Can you work these out from the model? Positions are in its coordinate system, mm. A direction names the side the tool comes from. Coordinates: 2 decimals unless noted, no trailing zeros. Loops run counter-clockwise (first coordinate to the right, second up) from the corner with the lowest first, then second, coordinate; pieces in that order, holes last. Notation, with made-up numbers: M 57.5,27 L 74.5,27 A11 cw 74.5,47 Z; hole C 33.25,70 d6. An arc over 180 degrees is marked long. Return JSON: item names as keys, results as strings. Group by question number.
```python
from build123d import *

# Parameters (mm, degrees)
SKETCH1_W           = 30
SKETCH1_H           = 30
SKETCH1_W_2         = 26
SKETCH1_H_2         = 26
BOSS_EXTRUDE1_DEPTH = 800
SKETCH2_W           = 30
SKETCH2_H           = 30
SKETCH2_R           = 11
BOSS_EXTRUDE2_DEPTH = 10
BOSS_EXTRUDE3_START = -10
SKETCH3_W           = 30
SKETCH3_H           = 30
SKETCH3_R           = 11
BOSS_EXTRUDE3_DEPTH = 10
SKETCH4_R           = 11
CUT_EXTRUDE1_DEPTH  = 50


with BuildPart() as part:
    # Sketch1 → Boss-Extrude1 (new body)
    with BuildSketch(Plane.XY):
        Rectangle(SKETCH1_W, SKETCH1_H)
        Rectangle(SKETCH1_W_2, SKETCH1_H_2, mode=Mode.SUBTRACT)
    extrude(amount=BOSS_EXTRUDE1_DEPTH)

    # Sketch2 → Boss-Extrude2 (add)
    with BuildSketch(Plane(origin=(0, 0, 0), x_dir=(-1, 0, 0), z_dir=(0, 0, -1))):
        with Locations((0, 30)):
            Rectangle(SKETCH2_W, SKETCH2_H)
        with Locations((0, 30)):
            Circle(SKETCH2_R, mode=Mode.SUBTRACT)
    extrude(amount=-BOSS_EXTRUDE2_DEPTH)

    # Sketch3 → Boss-Extrude3 (add)
    with BuildSketch(Plane.XY.offset(800).offset(BOSS_EXTRUDE3_START)):
        with Locations((0, 30)):
            Rectangle(SKETCH3_W, SKETCH3_H)
        with Locations(Location((0, 30, 0), (0, 0, 180))):
            Circle(SKETCH3_R, mode=Mode.SUBTRACT)
    extrude(amount=BOSS_EXTRUDE3_DEPTH)

    # Sketch4 → Cut-Extrude1 (cut)
    with BuildSketch(Plane.XZ.offset(15)):
        with Locations(Location((0, 400, 0), (0, 0, 270))):
            Circle(SKETCH4_R)
    extrude(amount=-CUT_EXTRUDE1_DEPTH, mode=Mode.SUBTRACT)


solid = part.part
```
1) For pin 1 (6 mm diameter, centred on x = -9, y = 34.5, fed in from +Z); pin 2 (9 mm diameter, centred on x = 0, y = 24.5, fed in from +Z); pin 3 (12 mm diameter, centred on x = -8.5, z = 528, fed in from +Y), each with a flat end and sliding along its axis, tell me the tip position at first contact or that it passes through.
2) Suppose I cut it at C-C, the plane z = 400. List the corners of the cut face in (x, y) for me.
3) If we mould it in two halves opening along X, with no side actions, what happens to faces 4 (the face through (-10, 15, 395)), 5 (the face through (-15, 1, 394)), 6 (the face through (15, 1, 394)), 7 (the face through (2.38, 19.26, 4.93))? For each: +X half, -X half, draft (parallel to the pull), parting line (faces both ways), or undercut.
4) If I drill on line 1 (Y direction, x = 0, z = 796.25); line 2 (Y direction, x = -0.5, z = 493.5), over which ranges is the centre line in solid material (lowest first)? Write a range as from..to.
5) Suppose I cut it at A-A, the plane z = 718. List the corners of the cut face in (x, y) for me, then the cut area to 3 significant figures.
6) Suppose I cut it at D-D, the plane x = 0. List the corners of the cut face in (y, z) for me, then the cut area to 3 significant figures.
7) For faces 1 (the face through (0, -14, 411)), 2 (the face through (13, 0, 394)), 3 (the face through (-7, 40, 790)), which set-ups out of +Z, -Z, +X, -X, +Y, -Y let a thin tool reach every point of the face, with its end or its side?
8) Suppose I cut it at B-B, the plane y = 6.5. List the corners of the cut face in (x, z) for me, then the cut area to 3 significant figures.
Returned:
{
 "1": {"pin 1": "stops at z = 800", "pin 2": "passes through", "pin 3": "stops at y = 15"},
 "2": {"outline": "M -15,-15 L -11,-15 L -11,-13 L -13,-13 L -13,13 L -11,13 L -11,15 L -15,15 Z; M 11,-15 L 15,-15 L 15,15 L 11,15 L 11,13 L 13,13 L 13,-13 L 11,-13 Z"},
 "3": {"face 4": "draft", "face 5": "-X half", "face 6": "+X half", "face 7": "undercut"},
 "4": {"line 1": "y = -15..-13, 13..19, 41..45", "line 2": "y = -15..-13, 13..15"},
 "5": {"outline": "M -15,-15 L 15,-15 L 15,15 L -15,15 Z; hole M -13,-13 L 13,-13 L 13,13 L -13,13 Z", "area": "224 mm²"},
 "6": {"outline": "M -15,0 L -13,0 L -13,389 L -15,389 Z; M -15,411 L -13,411 L -13,800 L -15,800 Z; M 13,0 L 19,0 L 19,10 L 15,10 L 15,389 L 13,389 Z; M 13,411 L 15,411 L 15,790 L 19,790 L 19,800 L 13,800 Z; M 41,0 L 45,0 L 45,10 L 41,10 Z; M 41,790 L 45,790 L 45,800 L 41,800 Z", "area": "3,270 mm²"},
 "7": {"face 1": "+Y, -Y", "face 2": "+Z, -Z", "face 3": "+X, -X, +Y"},
 "8": {"outline": "M -15,0 L -13,0 L -13,800 L -15,800 Z; M 13,0 L 15,0 L 15,800 L 13,800 Z", "area": "3,200 mm²"}
}
